Read the model definition and answer for the solid it produces. Units are mm, in the model's axes. Round coordinates to 2 decimals unless told otherwise and drop trailing zeros. Loops run counter-clockwise (first coordinate to the right, second up) from the corner with the lowest first, then second, coordinate; pieces in that order, holes last. Notation, with made-up numbers: (-29, -12.5) -> (9, -12.5) arc R18 ccw to (9, 12.5) -> close; hole circle Ø8 at (71, 50). An arc over 180 degrees is marked (long way). Put each result on its own line as item: value.
from build123d import *

# Parameters (mm, degrees)
PAD_DEPTH    = 10
SKETCH001_R  = 1.5
POCKET_DEPTH = 10.001
CHAMFER_SIZE = 0.2


with BuildPart() as part:
    # Sketch → Pad (new body)
    with BuildSketch(Plane.XY):
        Polygon((2.8, 0), (1.4, 2.424871), (-1.4, 2.424871), (-2.8, 0), (-1.4, -2.424871), (1.4, -2.424871), align=None)
    extrude(amount=PAD_DEPTH)

    # Sketch001 (on Face8 of Pad) → Pocket (cut, through all)
    with BuildSketch(Plane.XY.offset(10)):
        Circle(SKETCH001_R)
    extrude(amount=-POCKET_DEPTH, mode=Mode.SUBTRACT)

    # Chamfer
    chamfer_edges = [part.edges().sort_by_distance(p)[0] for p in [
        (-1.5, 0, 10),
        (-1.5, 0, 0),
    ]]
    chamfer(chamfer_edges, length=CHAMFER_SIZE)


solid = part.part
Item 1: The part is cut by section A-A (x = 0). Determine the outline of the cut face in (y, z), then the cut area to 3 significant figures.
Derived:
outline: (-2.42, 0) -> (-1.7, 0) -> (-1.5, 0.2) -> (-1.5, 9.8) -> (-1.7, 10) -> (-2.42, 10) -> close; (1.5, 0.2) -> (1.7, 0) -> (2.42, 0) -> (2.42, 10) -> (1.7, 10) -> (1.5, 9.8) -> close
area: 18.4 mm^2
Item 2: Find the intervals of material crossed by line 1 along Y through (x, z) = (-0.1, 6.5); line 2 along X through (y, z) = (-0.4, 7); line 3 along X through (y, z) = (0.1, 9), in increasing order.
Derived:
line 1: y = -2.42 to -1.5, 1.5 to 2.42
line 2: x = -2.57 to -1.45, 1.45 to 2.57
line 3: x = -2.74 to -1.5, 1.5 to 2.74
Item 3: For a pull along X with two mould halves and no side action, classify faces 1 (the flat face through (-2.11, -1.195, 4.93)), 2 (the flat face through (0, -2.425, 5)), 3 (the cylindrical face through (-1.5, 0.07, 5.07)) as pulls with the +X half, pulls with the -X half, needs draft (parallel to the pull), parting line crosses it, or undercut.
Derived:
face 1: pulls with the -X half
face 2: needs draft
face 3: undercut
Item 4: Flat-ended cylindrical pins translate along their axes: pin 1 Ø1 at (x, z) = (-2, 6.5) entering from -Y; pin 2 Ø2 at (y, z) = (-0.5, 7.5) entering from +X; pin 3 Ø1 at (x, z) = (-1.5, 8) entering from +Y. Find the tip coordinate at first contact, or state that the pin passes through.
Derived:
pin 1: stops at y = -2.25
pin 2: stops at x = 2.8
pin 3: stops at y = 2.42
Item 5: The part is cut by section B-B (z = 2.5). Determine the outline of the cut face in (x, y), then the cut area to 3 significant figures.
Derived:
outline: (-2.8, 0) -> (-1.4, -2.42) -> (1.4, -2.42) -> (2.8, 0) -> (1.4, 2.42) -> (-1.4, 2.42) -> close; hole circle Ø3 at (0, 0)
area: 13.3 mm^2
